Autodesk Inventor part; units mm, degrees
ref_plane "YZ Plane" through (0, 0, 0) normal (1, 0, 0) x (0, 1, 0)
ref_plane "XZ Plane" through (0, 0, 0) normal (0, 1, 0) x (-1, 0, 0)
ref_plane "XY Plane" through (0, 0, 0) normal (0, 0, 1) x (1, 0, 0)
sketch "Эскиз1" plane through (0, 0, 0) normal (0, 1, 0) x (-1, 0, 0)
  arc A0 (-0.25, 9.2247) -> (0.25, 9.2247) centre (0, 8) ccw
  line L0 (-0.25, 10.9972) -> (-0.25, 9.2247)
  arc A1 (-0.25, 10.9972) -> (-1.1469, -10.94) centre (0, 0) ccw
  line L1 (-1.1469, -10.6297) -> (-1.1469, -10.94)
  line L2 (-0.8473, -10.6297) -> (-1.1469, -10.6297)
  line L3 (-0.8473, -10.9673) -> (-0.8473, -10.6297)
  arc A2 (-0.8473, -10.9673) -> (0.8535, -10.9668) centre (0, 0) ccw
  line L4 (0.8535, -10.6297) -> (0.8535, -10.9668)
  line L5 (1.1541, -10.6297) -> (0.8535, -10.6297)
  line L6 (1.1541, -10.9393) -> (1.1541, -10.6297)
  arc A3 (1.1541, -10.9393) -> (0.25, 10.9972) centre (0, 0) ccw
  line L7 (0.25, 9.2247) -> (0.25, 10.9972)
  circle A4 centre (8, 0) radius 1.25
  circle A5 centre (0, -8) radius 1.25
  circle A6 centre (-8, 0) radius 1.25
  circle A7 centre (0, -5.5) radius 0.75
  circle A8 centre (4.7631, 2.75) radius 0.75
  circle A9 centre (-4.7631, 2.75) radius 0.75
  circle A10 centre (0, 0) radius 2.9
  arc A11 (0.25, 9.2247) -> (-0.25, 9.2247) centre (0, 8) ccw
  circle A12 centre (0, 0) radius 26.5
  point P0 (0, 0)
  dimension "d3" = 53
extrude "Выдавливание1" add sketch "Эскиз1" along normal blind 3 contours A0 L7 A3 L6 L5 L4 A2 L3 L2 L1 A1 L0 | A12
sketch "Эскиз2" plane through (0, 3, 0) normal (0, 1, 0) x (1, 0, 0)
  arc A0 (-14.8717, -1.6857) -> (-18.0997, 0.0968) centre (-15.9998, 0.0856) ccw
  arc A1 (-6.8718, -1.7285) -> (-9.1468, -1.7163) centre (-7.9999, 0.0428) ccw
  circle A2 centre (0, 0) radius 4
  arc A3 (-1.7285, 6.8718) -> (-1.7163, 9.1468) centre (0.0428, 7.9999) ccw
  arc A4 (-1.6857, 14.8717) -> (0.0968, 18.0997) centre (0.0856, 15.9998) ccw
  arc A5 (6.8718, 1.7285) -> (9.1468, 1.7163) centre (7.9999, -0.0428) ccw
  arc A6 (14.8717, 1.6857) -> (18.0997, -0.0968) centre (15.9998, -0.0856) ccw
  arc A7 (1.7285, -6.8718) -> (1.7163, -9.1468) centre (-0.0428, -7.9999) ccw
  arc A8 (1.6857, -14.8717) -> (-0.0968, -18.0997) centre (-0.0856, -15.9998) ccw
  circle A9 centre (-15.9998, 0.0856) radius 2.1
  circle A10 centre (-7.9999, 0.0428) radius 2.1
  circle A11 centre (0, 0) radius 4
  circle A12 centre (0.0428, 7.9999) radius 2.1
  circle A13 centre (0.0856, 15.9998) radius 2.1
  circle A14 centre (7.9999, -0.0428) radius 2.1
  circle A15 centre (15.9998, -0.0856) radius 2.1
  circle A16 centre (-0.0428, -7.9999) radius 2.1
  circle A17 centre (-0.0856, -15.9998) radius 2.1
  dimension "d4" = 4.2
extrude "Выдавливание2" cut sketch "Эскиз2" against normal blind 10 contours A9 A0 | A13 A4 | A15 A6 | A17 A8
properties part number "КВ33.044.405 -  Боковина шкива"
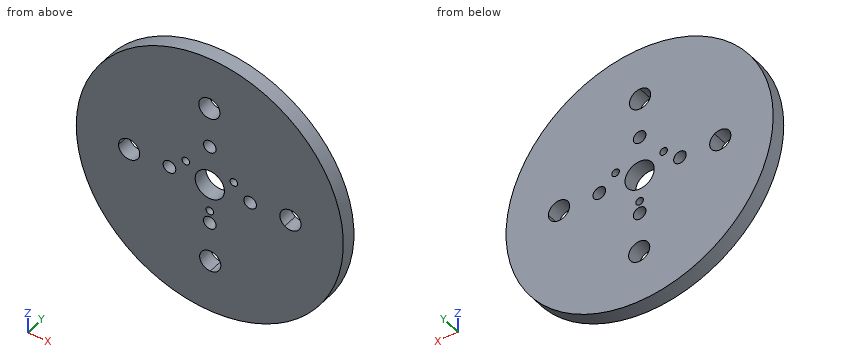
Geometry check sheet. Reference: the model listing, model coordinates, mm. Round coordinates to 2 decimals unless told otherwise and drop trailing zeros. Loops run counter-clockwise (first coordinate to the right, second up) from the corner with the lowest first, then second, coordinate; pieces in that order, holes last. Notation, with made-up numbers: (34.25, -16.75) - (39.25, -16.75) arc R22 cw to (39.25, 13.25) - close; hole circle Ø1 at (-27, -37). An arc over 180 degrees is marked (long way). One line per question, with ' | ' between items. Start each with the question number.
1. Scan lines: line 1 (X direction, y = 0.4, z = -0.5); line 2 (X direction, y = 0.8, z = 8); line 3 (X direction, y = 0.75, z = 16). Record each from-to range of solid material in increasing order. Write a range as [from, to].
2. Cross-section at B-B on x = -8. Record the cut outline in (y, z), then the cut area to 3 significant figures.
3. Depth check by flat-ended pin: pin 1 (0.9 mm diameter, centred on x = -4.76, z = 2.75, fed in from +Y). Enter the tip coordinate at first touch or a pass-through.
4. Cross-section at C-C on y = 0.95. State how many separate pieces and enclosed holes the cut face has, then the cut area to 3 significant figures.
5. Cross-section at D-D on z = -20.5. Record the cut outline in (x, y), then the cut area to 3 significant figures.
6. Cross-section at A-A on z = -5.5. Record the cut outline in (x, y).
Taken from the geometry:
1) line 1: [-26.5, -18.06], [-13.94, -9.15], [-6.85, -2.86], [2.86, 6.85], [9.15, 13.98], [18.02, 26.5] | line 2: [-25.26, -1.25], [1.25, 25.26] | line 3: [-21.12, -2.19], [2.01, 21.12]
2) outline: (0, -25.26) - (3, -25.26) - (3, -1.25) - (0, -1.25) - close; (0, 1.25) - (3, 1.25) - (3, 25.26) - (0, 25.26) - close | area: 144 mm²
3) pin 1: through
4) separate pieces: 1 | enclosed holes: 12 | area: 2,100 mm²
5) outline: (-16.79, 0) - (16.79, 0) - (16.79, 3) - (-16.79, 3) - close | area: 101 mm²
6) outline: (-25.92, 0) - (-0.75, 0) - (-0.75, 3) - (-25.92, 3) - close; (0.75, 0) - (25.92, 0) - (25.92, 3) - (0.75, 3) - close
